Geometry check sheet. Reference: the model listing, model coordinates, mm. A direction names the side the tool comes from. Coordinates: 2 decimals unless noted, no trailing zeros. Order: outer loops, then holes, each group sorted by start corner. A loop starts at its lowest first (then second) coordinate and runs counter-clockwise, first axis right, second up. Notation, with made-up numbers: (43, 65.5) -> (96, 65.5) arc R36 cw to (96, 103.5) -> close; hole circle Ø1 at (79, -12). An arc over 180 degrees is marked (long way). Answer as CSV lines item,"result". Start each with the question number.
from build123d import *

# Parameters (mm, degrees)
SKETCH_R     = 5
PAD_DEPTH    = 5
PAD001_DEPTH = 2.5
FILLET_R     = 5
CHAMFER_SIZE = 1


with BuildPart() as part:
    # Sketch → Pad (new body)
    with BuildSketch(Plane.XY):
        with BuildLine():
            Line((-50, 20), (-50, -20))
            ThreePointArc((-50, -20), (-48.535534, -23.535534), (-45, -25))
            Line((-45, -25), (45, -25))
            ThreePointArc((45, -25), (48.535534, -23.535534), (50, -20))
            Line((50, -20), (50, 20))
            ThreePointArc((50, 20), (48.535534, 23.535534), (45, 25))
            Line((45, 25), (-45, 25))
            ThreePointArc((-45, 25), (-48.535534, 23.535534), (-50, 20))
        make_face()
        with Locations((-40, 15)):
            Circle(SKETCH_R, mode=Mode.SUBTRACT)
        with Locations((40, 15)):
            Circle(SKETCH_R, mode=Mode.SUBTRACT)
        with Locations((40, -15)):
            Circle(SKETCH_R, mode=Mode.SUBTRACT)
        with Locations((-40, -15)):
            Circle(SKETCH_R, mode=Mode.SUBTRACT)
    extrude(amount=PAD_DEPTH)

    # Sketch001 → Pad001 (join, symmetric)
    with BuildSketch(Plane.XZ):
        with BuildLine():
            Line((-30, 30), (30, 30))
            ThreePointArc((50, 10), (44.142136, 24.142136), (30, 30))
            Line((50, 10), (50, 5))
            Line((50, 5), (-50, 5))
            Line((-50, 5), (-50, 10))
            ThreePointArc((-30, 30), (-44.142136, 24.142136), (-50, 10))
        make_face()
    extrude(amount=PAD001_DEPTH, both=True)

    # Fillet
    fillet_edges = [part.edges().sort_by_distance(p)[0] for p in [
        (0, -2.5, 5),
        (0, 2.5, 5),
    ]]
    fillet(fillet_edges, radius=FILLET_R)

    # Chamfer
    chamfer_edges = [part.edges().sort_by_distance(p)[0] for p in [
        (35, -15, 5),
        (-45, -15, 5),
        (-45, 15, 5),
        (35, 15, 5),
    ]]
    chamfer(chamfer_edges, length=CHAMFER_SIZE)


solid = part.part
Q1. Sectioned sample at D-D, the plane x = 40. Record the cut outline in (y, z), then the cut area to 3 significant figures.
Q2. Sectioned sample at A-A, the plane y = 15. Record the cut outline in (x, z), then the cut area to 3 significant figures.
Q3. Go/stop test with flat-tipped pins: pin 1 Ø9 at (x, y) = (16, 15) entering from +Z; pin 2 Ø5 at (y, z) = (0, 20) entering from +X; pin 3 Ø5 at (x, z) = (12.5, 23) entering from -Y. Record where each tip stops, or that it passes through.
Q4. Release check for a two-part mould opening along Y. For faces 3 (the cylindrical face through (36, 12, 2)), 4 (the cylindrical face through (-45, -15, 2)), 5 (the flat face through (-1, -16, 5)), 6 (the flat face through (1, 2.5, 20)) record: released by +Y, released by -Y, zero draft, split by the parting line, or undercut.
Q5. Thickness scan on L1, parallel to Y at x = -40, z = 1; L2, parallel to Y at x = 4, z = 25; L3, parallel to Z at x = 35, y = 23.5. Record the ranges inside material, lowest first.
Q6. Sectioned sample at C-C, the plane y = 1.5. Record the cut outline in (x, z).
Q7. Access from +Z, -Z, +X, -X, +Y, -Y to the whole of each face (thin tool, end or side, straight path). Record for faces 1 (the flat face through (0, 0, 30)), 2 (the flat face through (-1, 16, 5)).
Q8. Sectioned sample at B-B, the plane x = 20. Record the cut outline in (y, z), then the cut area to 3 significant figures.
Geometry results:
1,outline,"(-25, 0) -> (-20, 0) -> (-20, 4) -> (-21, 5) -> (-25, 5) -> close; (-10, 0) -> (10, 0) -> (10, 4) -> (9, 5) -> (7.5, 5) arc R5 cw to (2.5, 10) -> (2.5, 27.32) -> (-2.5, 27.32) -> (-2.5, 10) arc R5 cw to (-7.5, 5) -> (-9, 5) -> (-10, 4) -> close; (20, 0) -> (25, 0) -> (25, 5) -> (21, 5) -> (20, 4) -> close"
1,area,"270 mm^2"
2,outline,"(-50, 0) -> (-45, 0) -> (-45, 4) -> (-46, 5) -> (-50, 5) -> close; (-35, 0) -> (35, 0) -> (35, 4) -> (34, 5) -> (-34, 5) -> (-35, 4) -> close; (45, 0) -> (50, 0) -> (50, 5) -> (46, 5) -> (45, 4) -> close"
2,area,"398 mm^2"
3,pin 1,"stops at z = 5"
3,pin 2,"stops at x = 48.54"
3,pin 3,"stops at y = -2.5"
4,face 3,"undercut"
4,face 4,"undercut"
4,face 5,"zero draft"
4,face 6,"released by +Y"
5,L1,"y = -25 to -20, -10 to 10, 20 to 25"
5,L2,"y = -2.5 to 2.5"
5,L3,"z = 0 to 5"
6,outline,"(-50, 0) -> (50, 0) -> (50, 10) arc R20 ccw to (30, 30) -> (-30, 30) arc R20 ccw to (-50, 10) -> close"
7,face 1,"+Z, +X, -X, +Y, -Y"
7,face 2,"+Z, +X, -X, +Y"
8,outline,"(-25, 0) -> (25, 0) -> (25, 5) -> (7.5, 5) arc R5 cw to (2.5, 10) -> (2.5, 30) -> (-2.5, 30) -> (-2.5, 10) arc R5 cw to (-7.5, 5) -> (-25, 5) -> close"
8,area,"386 mm^2"
